For this review, take the finished solid that the model builds, in its own axes (mm). A direction names the side the tool comes from. Coordinates: 2 decimals unless noted, no trailing zeros. Write each loop counter-clockwise with the first axis right and the second up, starting at its lowest first coordinate (ties: lowest second). Pieces come first, ordered by that corner, then holes. Notation, with made-up numbers: (32.5, 4) -> (48.5, 4) arc R23 cw to (48.5, 33) -> close; hole circle Ø8 at (25, 16.5). An arc over 180 degrees is marked (long way). One line per item, written item: value. Start each with the question number.
1) Add section C-C (x = -5). State the section outline as (y, z) points.
2) For pin 1 Ø1.8 at (y, z) = (1, -13.5) entering from -X; pin 2 Ø1.8 at (y, z) = (-0.5, 26) entering from +X; pin 3 Ø0.6 at (x, y) = (-5, 1.5) entering from -Z; pin 4 Ø1.5 at (y, z) = (2.5, -4.5) entering from +X, all flat-tipped, find the tip position at first contact; note any pin that passes through.
3) Machinability: for faces 1 (the cylindrical face through (-2.815, -0.042, 20.301)), 2 (the cylindrical face through (2.97, -0.04, 14.4)), 3 (the flat face through (-5, 0, 15)), which of the approach directions +Z, -Z, +X, -X, +Y, -Y give a long, thin tool a straight path to every point of the face, cutting with its end or side? Answer none if there is none.
4) Mouldability with a two-part tool opening along Y and no side actions: class faces 4 (the cylindrical face through (-5.269, 2.715, 29.699)), 5 (the flat face through (5, 0, 30)), 6 (the cylindrical face through (-5.27, 0.07, 27.5)) as released by +Y, released by -Y, zero draft, split by the parting line, or undercut.
5) Add section A-A (y = 0). State how many separate pieces and enclosed holes the cut face has, and give its area (3 significant figures).
6) Add section B-B (z = 26). State the section outline as (x, y) points, and give its area (3 significant figures).
7) Add section D-D (z = -25.5). State the section outline as (x, y) points.
8) For probe 1 along Y at (x, z) = (4.5, 26); probe 2 along X at (y, z) = (-1.65, 25); probe 3 along X at (y, z) = (-1.55, -22), list the stretches that pass through material, from the lowest coordinate up. Write a range as from..to.
from build123d import *
from build123d.topology import SkipClean

# Parameters (mm, degrees)
SALIENTE_EXTRUIR1_DEPTH    = 2.4
CORTAR_EXTRUIR1_DEPTH      = 31.244999587
CORTAR_EXTRUIR1_DEPTH_BACK = 31.244999587
CROQUIS2_R                 = 1.5
CROQUIS3_R                 = 1.5
SALIENTE_EXTRUIR2_DEPTH    = 7.5
CORTAR_EXTRUIR2_DEPTH      = 3.1
REDONDEO1_R                = 2
REDONDEO2_R                = 1


with BuildPart() as part:
    # Croquis1 → Saliente-Extruir1 (new, symmetric)
    with BuildSketch(Plane(origin=(0, 0, 0), x_dir=(0, 0, -1), z_dir=(1, 0, 0))):
        with BuildLine():
            Line((-29, 3), (29, 3))
            ThreePointArc((29, 3), (29.707106781, 2.707106781), (30, 2))
            Line((30, 2), (30, -2))
            ThreePointArc((30, -2), (29.707106781, -2.707106781), (29, -3))
            Line((29, -3), (-29, -3))
            ThreePointArc((-29, -3), (-29.707106781, -2.707106781), (-30, -2))
            Line((-30, -2), (-30, 2))
            ThreePointArc((-30, 2), (-29.707106781, 2.707106781), (-29, 3))
        make_face()
    extrude(amount=SALIENTE_EXTRUIR1_DEPTH, both=True)

    # Croquis2 → Cortar-Extruir1 (cut, two sides: drawn at the far end of the back side and taken through both)
    with BuildSketch(Plane(origin=(0, 0, 0), x_dir=(0, 0, -1), z_dir=(1, 0, 0)).offset(-CORTAR_EXTRUIR1_DEPTH_BACK)):
        with Locations((-26, 0)):
            Circle(CROQUIS2_R)
        with Locations((26, 0)):
            Circle(CROQUIS2_R)
    extrude(amount=CORTAR_EXTRUIR1_DEPTH + CORTAR_EXTRUIR1_DEPTH_BACK, mode=Mode.SUBTRACT)

    # Croquis3 → Saliente-Extruir2 (add, symmetric)
    with SkipClean():  # the faces are left unmerged after this step: merging them gives an invalid solid
        with BuildSketch(Plane(origin=(0, 0, 0), x_dir=(0, 0, -1), z_dir=(1, 0, 0))):
            with BuildLine():
                Line((-30, 2), (-30, -2))
                ThreePointArc((-30, -2), (-29.707106781, -2.707106781), (-29, -3))
                Line((-29, -3), (-15, -3))
                Line((-15, -3), (-15, 3))
                Line((-15, 3), (-29, 3))
                ThreePointArc((-29, 3), (-29.707106781, 2.707106781), (-30, 2))
            make_face()
            with Locations((-26, 0)):
                Circle(CROQUIS3_R, mode=Mode.SUBTRACT)
        extrude(amount=SALIENTE_EXTRUIR2_DEPTH, both=True)
    add(part.part.scale(1), mode=Mode.REPLACE)  # the faces are merged on a copy

    # Croquis4 → Cortar-Extruir2 (cut, symmetric)
    with BuildSketch(Plane(origin=(0, 0, 0), x_dir=(0, 0, -1), z_dir=(1, 0, 0))):
        with BuildLine():
            Line((-29, 3), (-20, 3))
            Line((-20, 3), (-20, -3))
            Line((-20, -3), (-29, -3))
            ThreePointArc((-29, -3), (-29.707106781, -2.707106781), (-30, -2))
            Line((-30, -2), (-30, 2))
            ThreePointArc((-30, 2), (-29.707106781, 2.707106781), (-29, 3))
        make_face()
    extrude(amount=CORTAR_EXTRUIR2_DEPTH, both=True, mode=Mode.SUBTRACT)

    # Redondeo1
    redondeo1_edges = [part.edges().sort_by_distance(p)[0] for p in [
        (-2.4, 0, 15),
        (2.4, 0, 15),
        (-7.5, 0, 15),
        (7.5, 0, 15),
    ]]
    fillet(redondeo1_edges, radius=REDONDEO1_R)

    # Redondeo2
    redondeo2_edges = [part.edges().sort_by_distance(p)[0] for p in [
        (3.1, 0, 20),
        (-3.1, 0, 20),
    ]]
    fillet(redondeo2_edges, radius=REDONDEO2_R)


solid = part.part
Numbers:
1. outline: (-3, 15) -> (3, 15) -> (3, 29) arc R1 ccw to (2, 30) -> (-2, 30) arc R1 ccw to (-3, 29) -> close; hole circle Ø3 at (0, 26)
2. pin 1: x = -2.4
2. pin 2: through
2. pin 3: z = 15
2. pin 4: x = 2.4
3. face 1: +Z, +Y, -Y
3. face 2: -Z, +X, +Y, -Y
3. face 3: -Z, -X, +Y, -Y
4. face 4: released by +Y
4. face 5: zero draft
4. face 6: undercut
5. separate pieces: 4
5. enclosed holes: 0
5. area: 339 mm²
6. outline: (-7.5, -3) -> (-3.1, -3) -> (-3.1, -1.5) -> (-7.5, -1.5) -> close; (-7.5, 1.5) -> (-3.1, 1.5) -> (-3.1, 3) -> (-7.5, 3) -> close; (3.1, -3) -> (7.5, -3) -> (7.5, -1.5) -> (3.1, -1.5) -> close; (3.1, 1.5) -> (7.5, 1.5) -> (7.5, 3) -> (3.1, 3) -> close
6. area: 26.4 mm²
7. outline: (-2.4, -3) -> (2.4, -3) -> (2.4, -1.41) -> (-2.4, -1.41) -> close; (-2.4, 1.41) -> (2.4, 1.41) -> (2.4, 3) -> (-2.4, 3) -> close
8. probe 1: -3..-1.5, 1.5..3
8. probe 2: -7.5..-3.1, 3.1..7.5
8. probe 3: -2.4..2.4
